from build123d import *

# Parameters (mm, degrees)
SKETCH1_R           = 30
SKETCH1_R_2         = 25
BOSS_EXTRUDE1_DEPTH = 145
SKETCH2_R           = 25
BOSS_EXTRUDE2_DEPTH = 10
SKETCH3_R           = 25
BOSS_EXTRUDE3_DEPTH = 10
SKETCH11_R          = 30
SKETCH11_R_2        = 28.945980101
CUT_EXTRUDE2_DEPTH  = 10
SKETCH12_R          = 30
SKETCH12_R_2        = 29.420954363
CUT_EXTRUDE3_DEPTH  = 10


with BuildPart() as part:
    # Sketch1 → Boss-Extrude1 (new body)
    with BuildSketch(Plane.XY):
        Circle(SKETCH1_R)
        Circle(SKETCH1_R_2, mode=Mode.SUBTRACT)
    extrude(amount=BOSS_EXTRUDE1_DEPTH)

    # Sketch2 → Boss-Extrude2 (add)
    with BuildSketch(Plane.XY):
        Circle(SKETCH2_R)
    extrude(amount=BOSS_EXTRUDE2_DEPTH)

    # Sketch3 → Boss-Extrude3 (add)
    with BuildSketch(Plane.XY.offset(135)):
        Circle(SKETCH3_R)
    extrude(amount=BOSS_EXTRUDE3_DEPTH)

    # Sketch11 → Cut-Extrude2 (cut)
    with BuildSketch(Plane(origin=(0, 0, 0), x_dir=(-1, 0, 0), z_dir=(0, 0, -1))):
        Circle(SKETCH11_R)
        Circle(SKETCH11_R_2, mode=Mode.SUBTRACT)
    extrude(amount=-CUT_EXTRUDE2_DEPTH, mode=Mode.SUBTRACT)

    # Sketch12 → Cut-Extrude3 (cut)
    with BuildSketch(Plane.XY.offset(145)):
        Circle(SKETCH12_R)
        Circle(SKETCH12_R_2, mode=Mode.SUBTRACT)
    extrude(amount=-CUT_EXTRUDE3_DEPTH, mode=Mode.SUBTRACT)


solid = part.part
Input: part model. Units: mm. Frame: model coordinates. A direction names the side the tool comes from. Coordinates: 2 decimals unless noted, no trailing zeros. Loops run counter-clockwise (first coordinate to the right, second up) from the corner with the lowest first, then second, coordinate; pieces in that order, holes last. Notation, with made-up numbers: (81, 87.5) -> (120, 87.5) arc R23 cw to (120, 115.5) -> close; hole circle Ø8 at (72.5, 21.25). An arc over 180 degrees is marked (long way). Write each question's results on one line, items separated by ' | '. Start each with the question number.
Q1. Section A-A, the plane x = 0. Return the cut outline in (y, z), plus the area to 3 significant figures.
Q2. Section C-C, the plane z = 58. Return the cut outline in (x, y).
Q3. Pull-direction query (Y, two-part tool) for faces 1 (the flat face through (0, 0, 10)), 2 (the cylindrical face through (-3.83, 29.17, 140.07)), 3 (the flat face through (16, 25, 10)); classes: released by +Y, released by -Y, zero draft, split by the parting line, or undercut.
Q4. Pin query (flat end, axial travel): pin 1 (6 mm diameter, centred on y = 19, z = 22, fed in from +X); pin 2 (1.5 mm diameter, centred on y = -24, z = 72, fed in from +X); pin 3 (3 mm diameter, centred on y = 10.5, z = 100.5, fed in from -X). Return the tip coordinate at first contact, or that it passes through.
Q5. Ray query, line 1 (Y direction, x = 0, z = 90); line 2 (Z direction, x = 13, y = -3); line 3 (X direction, y = 8, z = 103.5). Return the intervals inside material, ascending. Write a range as from..to.
Q6. Reachability of faces 4 (the cylindrical face through (-27.61, 8.69, 4.93)), 5 (the cylindrical face through (23.846, 7.509, 71.625)), 6 (the flat face through (22, -20, 135)) from +Z, -Z, +X, -X, +Y, -Y: full face, straight path, thin tool, end or side. Return the list, or none.
Found:
1) outline: (-30, 10) -> (-28.95, 10) -> (-28.95, 0) -> (28.95, 0) -> (28.95, 10) -> (30, 10) -> (30, 135) -> (29.42, 135) -> (29.42, 145) -> (-29.42, 145) -> (-29.42, 135) -> (-30, 135) -> close; hole (-25, 10) -> (25, 10) -> (25, 135) -> (-25, 135) -> close | area: 2,420 mm2
2) outline: circle Ø60 at (0, 0); hole circle Ø50 at (0, 0)
3) face 1: undercut | face 2: split by the parting line | face 3: zero draft
4) pin 1: x = 25.38 | pin 2: x = 18.96 | pin 3: x = -28.62
5) line 1: -30..-25, 25..30 | line 2: 0..10, 135..145 | line 3: -28.91..-23.69, 23.69..28.91
6) face 4: -Z | face 5: none | face 6: +Z
